Part print with two shaded views. Sizes in mm from the minimum x, y, z corner. A direction names the side the tool comes from. Round coordinates to 2 decimals unless told otherwise and drop trailing zeros. Write each loop counter-clockwise with the first axis right and the second up, starting at its lowest first coordinate (ties: lowest second). Pieces come first, ordered by that corner, then holes.
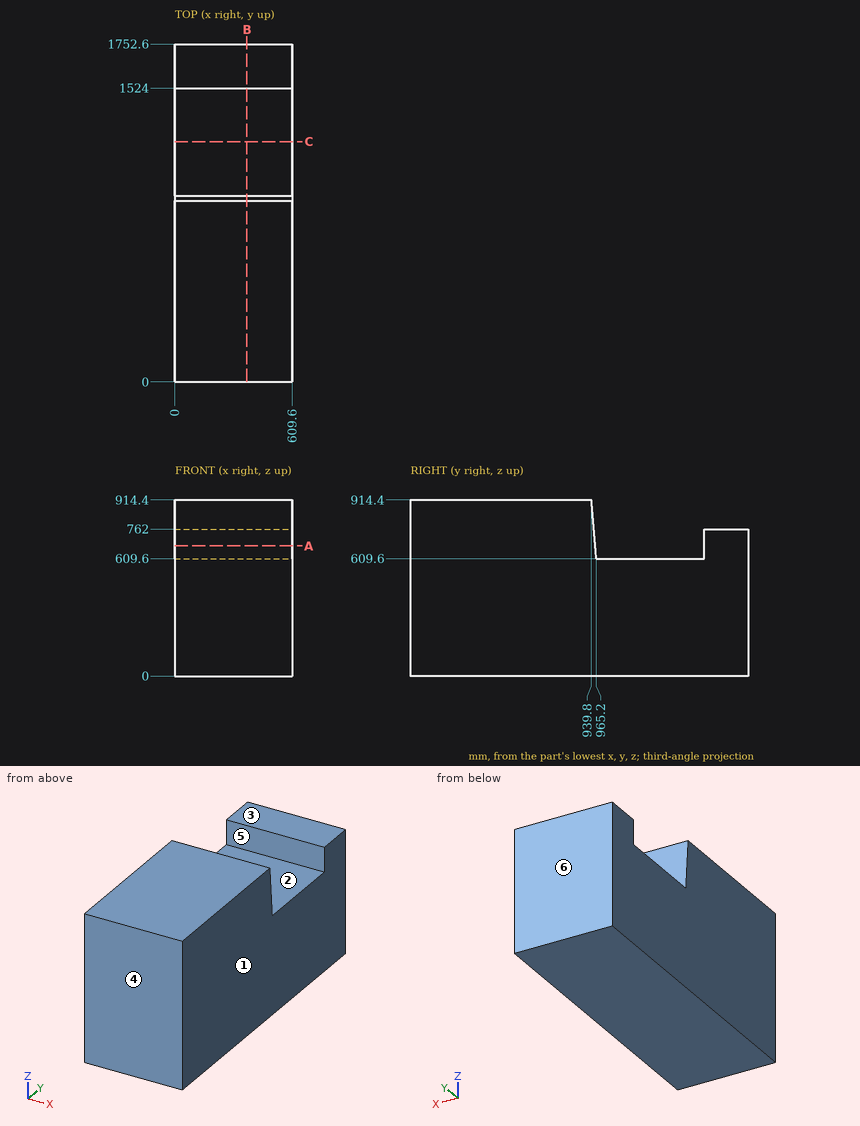
Q1. Which spindle directions (+Z, -Z, +X, -X, +Y, -Y) get a long thin tool onto all of the face, cutting with end or side? Do the marked faces 1, 2 and 3. Say none if no direction does.
Values follow:
face 1: +Z, -Z, +X, +Y, -Y
face 2: +Z, +X, -X
face 3: +Z, +X, -X, +Y
Q2. Cut at C-C on y = 1245.5. Write the cut outline in (x, z).
Values follow:
outline: (0, 0) - (609.6, 0) - (609.6, 609.6) - (0, 609.6) - close
Q3. Cut at B-B on x = 373. Write the cut outline in (y, z).
Values follow:
outline: (0, 0) - (1752.6, 0) - (1752.6, 762) - (1524, 762) - (1524, 609.6) - (965.2, 609.6) - (939.8, 914.4) - (0, 914.4) - close
Q4. Wall check: L1, parallel to Z at x = 414, y = 1116.5; L2, parallel to Y at x = 445.5, z = 793; L3, parallel to Y at x = 402.5, z = 786. Give the ranges that are in metal, low to high.
Values follow:
L1: z = 0 to 609.6
L2: y = 0 to 949.92
L3: y = 0 to 950.5
Q5. Cut at A-A on z = 675. Write the cut outline in (x, y), plus the area to 3 significant figures.
Values follow:
outline: (0, 0) - (609.6, 0) - (609.6, 959.75) - (0, 959.75) - close; (0, 1524) - (609.6, 1524) - (609.6, 1752.6) - (0, 1752.6) - close
area: 724,000 mm2
Q6. Mould opens along Y. For the marked faces 4, 5 and 6 say: +Y half, -Y half, draft (parallel to the pull), parting line (faces both ways), or undercut.
Values follow:
face 4: -Y half
face 5: undercut
face 6: +Y half
